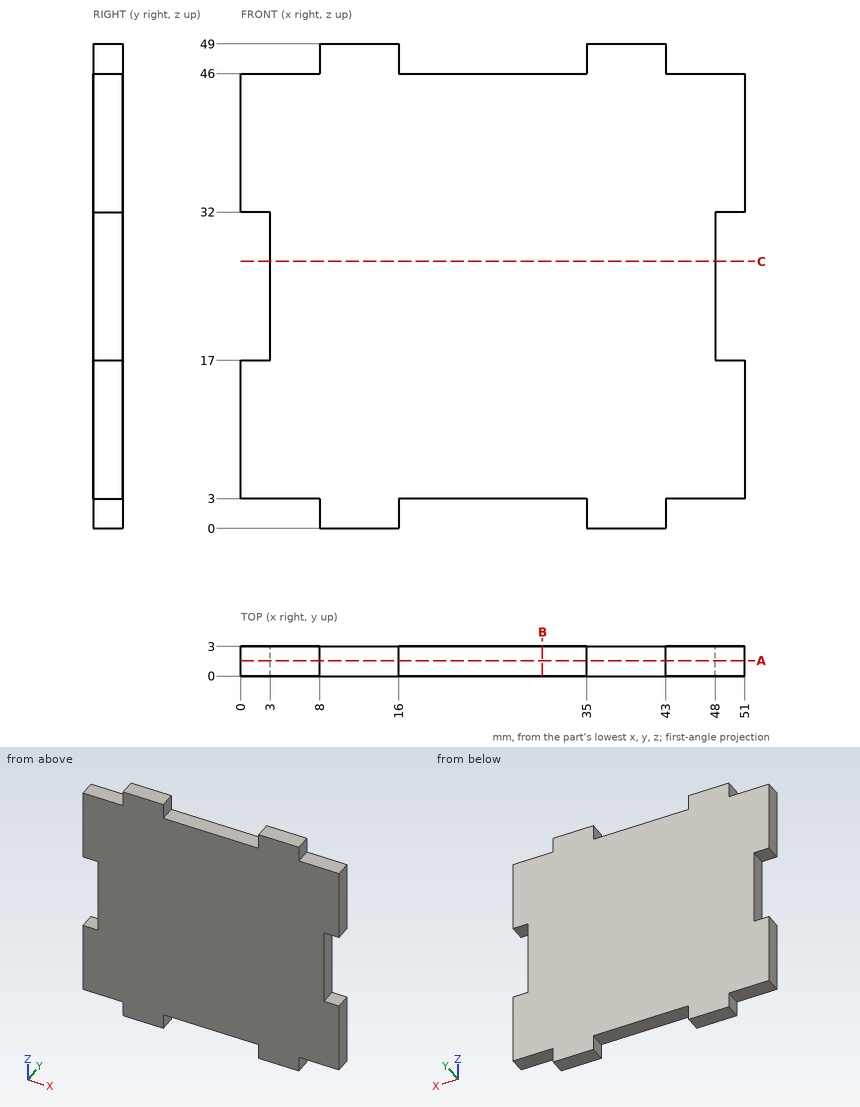
Verification items for this drawing (mm, ordinates from the low corner). Round coordinates to 2 decimals unless told otherwise and drop trailing zeros. Write each loop counter-clockwise with the first axis right and the second up, starting at its lowest first coordinate (ties: lowest second). Pieces come first, ordered by that corner, then holes. Notation, with made-up numbers: (65, 22.5) - (79, 22.5) arc R12 ccw to (79, 31.5) - close; hole circle Ø3 at (80, 48). An arc over 180 degrees is marked (long way). One line per item, written item: value.
1. Cross-section at C-C on z = 27. Record the boundary of the cut face in (x, y).
The answers:
outline: (3, 0) - (48, 0) - (48, 3) - (3, 3) - close
2. Cross-section at A-A on y = 1.55. Record the boundary of the cut face in (x, z), and give its area (3 significant figures).
The answers:
outline: (0, 3) - (8, 3) - (8, 0) - (16, 0) - (16, 3) - (35, 3) - (35, 0) - (43, 0) - (43, 3) - (51, 3) - (51, 17) - (48, 17) - (48, 32) - (51, 32) - (51, 46) - (43, 46) - (43, 49) - (35, 49) - (35, 46) - (16, 46) - (16, 49) - (8, 49) - (8, 46) - (0, 46) - (0, 32) - (3, 32) - (3, 17) - (0, 17) - close
area: 2,200 mm^2
3. Depth check by flat-ended pin: pin 1 Ø1.5 at (x, y) = (47, 1) entering from +Z; pin 2 Ø1.5 at (x, y) = (47.5, 1.5) entering from -Z; pin 3 Ø0.9 at (y, z) = (1, 48) entering from +X; pin 4 Ø1.5 at (x, z) = (40, 21.5) entering from -Y. Enter the tip coordinate at first touch or a pass-through.
The answers:
pin 1: stops at z = 46
pin 2: stops at z = 3
pin 3: stops at x = 43
pin 4: stops at y = 0
4. Cross-section at B-B on x = 30.5. Record the boundary of the cut face in (y, z), and give its area (3 significant figures).
The answers:
outline: (0, 3) - (3, 3) - (3, 46) - (0, 46) - close
area: 129 mm^2
5. Scan lines: L1, parallel to Z at x = 2, y = 0.2; L2, parallel to X at y = 0.5, z = 21; L3, parallel to X at y = 2.9, z = 46.5. Record each from-to range of solid material in increasing order.
The answers:
L1: z = 3 to 17, 32 to 46
L2: x = 3 to 48
L3: x = 8 to 16, 35 to 43
